```python
from build123d import *

# Parameters (mm, degrees)
SKETCH1_W               = 50
SKETCH1_H               = 100
BOSS_EXTRUDE1_DEPTH     = 90
CUT_EXTRUDE1_DEPTH      = 115.455231423
CUT_EXTRUDE1_DEPTH_BACK = 115.455231423
SKETCH2_R               = 3.2
CHAMFER1_SIZE           = 2
CUT_EXTRUDE2_START      = -5
SKETCH3_W               = 28.111922991
SKETCH3_H               = 15
CUT_EXTRUDE2_DEPTH      = 8
SKETCH4_R               = 4.125
CUT_EXTRUDE3_DEPTH      = 8
SKETCH6_W               = 5
SKETCH6_H               = 5
CUT_EXTRUDE4_DEPTH      = 108.964114408


with BuildPart() as part:
    # Sketch1 → Boss-Extrude1 (new body)
    with BuildSketch(Plane.YZ):
        Rectangle(SKETCH1_W, SKETCH1_H)
    extrude(amount=BOSS_EXTRUDE1_DEPTH)

    # Sketch2 → Cut-Extrude1 (cut, two sides: drawn at the far end of the back side and taken through both)
    with BuildSketch(Plane(origin=(0, 25, 0), x_dir=(-1, 0, 0), z_dir=(0, 1, 0)).offset(-CUT_EXTRUDE1_DEPTH_BACK)):
        with Locations(Location((-15, -25, 0), (0, 0, 90))):
            Circle(SKETCH2_R)
        with Locations(Location((-15, 25, 0), (0, 0, 270))):
            Circle(SKETCH2_R)
    extrude(amount=CUT_EXTRUDE1_DEPTH + CUT_EXTRUDE1_DEPTH_BACK, mode=Mode.SUBTRACT)

    # Chamfer1
    chamfer1_edges = [part.edges().sort_by_distance(p)[0] for p in [
        (45, 25, 50),
        (45, -25, 50),
        (0, 0, 50),
        (90, 0, 50),
        (45, 25, -50),
        (0, 25, 0),
        (90, 25, 0),
        (15, 25, -28.2),
        (15, 25, 28.2),
        (45, -25, -50),
        (15, -25, 28.2),
        (15, -25, -28.2),
        (0, 0, -50),
        (90, 0, -50),
    ]]
    chamfer(chamfer1_edges, length=CHAMFER1_SIZE)

    # Sketch3 → Cut-Extrude2 (cut)
    with BuildSketch(Plane.XY.offset(50).offset(CUT_EXTRUDE2_START)):
        Polygon((66.5, 7.5), (72.995190528, 3.75), (72.995190528, -3.75), (66.5, -7.5), (88, -7.5), (88, 7.5), align=None)
        with Locations((102.055961496, 0)):
            Rectangle(SKETCH3_W, SKETCH3_H)
        Polygon((66.5, -7.5), (72.995190528, -3.75), (72.995190528, 3.75), (66.5, 7.5), (60.004809472, 3.75), (60.004809472, -3.75), align=None)
    cut_extrude2 = extrude(amount=-CUT_EXTRUDE2_DEPTH, mode=Mode.SUBTRACT)

    # Sketch4 → Cut-Extrude3 (cut)
    with BuildSketch(Plane.XY.offset(50)):
        with Locations((66.5, 0)):
            Circle(SKETCH4_R)
    cut_extrude3 = extrude(amount=-CUT_EXTRUDE3_DEPTH, mode=Mode.SUBTRACT)

    # Sketch6 → Cut-Extrude4 (cut, symmetric)
    with BuildSketch(Plane.XZ.offset(-7.5)):
        with Locations((64, 39.5)):
            Rectangle(SKETCH6_W, SKETCH6_H)
    cut_extrude4 = extrude(amount=CUT_EXTRUDE4_DEPTH, both=True, mode=Mode.SUBTRACT)

    # Mirror1: Cut-Extrude2, Cut-Extrude3, Cut-Extrude4 across plane
    add(cut_extrude2.mirror(Plane.XY), mode=Mode.SUBTRACT)
    add(cut_extrude3.mirror(Plane.XY), mode=Mode.SUBTRACT)
    add(cut_extrude4.mirror(Plane.XY), mode=Mode.SUBTRACT)


solid = part.part
```
Build history of the part. All positions in model axes, mm. A direction names the side the tool comes from. Coordinates: 2 decimals unless noted, no trailing zeros. Order: outer loops, then holes, each group sorted by start corner. A loop starts at its lowest first (then second) coordinate and runs counter-clockwise, first axis right, second up. Notation, with made-up numbers: M -36.75,89.25 L -22.75,89.25 A27 cw -22.75,121.25 Z; hole C -29,-29.5 d8. An arc over 180 degrees is marked long. One line per question, with ' | ' between items. Start each with the question number.
1. Tool access for faces 4 (the face through (66.5, -16, -39)), 5 (the face through (62.485, -5.182, 42.834)), 6 (the face through (70.435, 1.239, 47.535)): list every direction of +Z, -Z, +X, -X, +Y, -Y with a clear straight run to the whole face (end or side of a thin tool).
2. Wall check: line 1 along Z through (x, y) = (70.5, -1.5); line 2 along X through (y, z) = (0, -47.85) (3 decimals); line 3 along Y through (x, z) = (69.5, -40.5). Give the ranges that are in metal, low to high. Write a range as [from, to].
3. Cut at C-C (x = 15). Write the cut outline in (y, z), plus the area to 3 significant figures.
4. Cut at A-A (y = 0). Write the cut outline in (x, z) (3 decimals).
5. Flat gauge pins, fed straight in: P1, Ø2, axis at y = 0.5, z = 42.5, coming from the +X side; P2, Ø7.5, axis at x = 66.5, y = 0, coming from the +Z side; P3, Ø7.5, axis at x = 15, z = 25, coming from the -Y side. Where does each tip first touch, or does it go through?
6. Cut at B-B (z = -25). Write the cut outline in (x, y).
7. Mould opens along X. For faces 1 (the face through (61.5, -15, -39)), 2 (the face through (78, 7.5, -41)), 3 (the face through (60.005, 0, -41)) say: +X half, -X half, draft (parallel to the pull), parting line (faces both ways), or undercut.
The answers:
1) face 4: +Y, -Y | face 5: +X | face 6: +Z
2) line 1: z = [-50, -45], [-37, 37], [45, 50] | line 2: x = [0, 62.375], [70.625, 90] | line 3: y = [-25, -7.5], [7.5, 25]
3) outline: M -25,-48 L -23,-50 L 23,-50 L 25,-48 L 25,-30.2 L 23,-28.2 L -23,-28.2 L -25,-30.2 Z; M -25,-19.8 L -23,-21.8 L 23,-21.8 L 25,-19.8 L 25,19.8 L 23,21.8 L -23,21.8 L -25,19.8 Z; M -25,30.2 L -23,28.2 L 23,28.2 L 25,30.2 L 25,48 L 23,50 L -23,50 L -25,48 Z | area: 4,340 mm2
4) outline: M 0,-48 L 2,-50 L 62.375,-50 L 62.375,-45 L 60.005,-45 L 60.005,-37 L 90,-37 L 90,37 L 60.005,37 L 60.005,45 L 62.375,45 L 62.375,50 L 2,50 L 0,48 Z; M 70.625,-50 L 88,-50 L 90,-48 L 90,-45 L 70.625,-45 Z; M 70.625,45 L 90,45 L 90,48 L 88,50 L 70.625,50 Z; hole C 15,-25 d6.4; hole C 15,25 d6.4
5) P1: stops at x = 60 | P2: stops at z = 37 | P3: stops at y = -23.55
6) outline: M 0,-25 L 9.8,-25 L 11.8,-23 L 11.8,23 L 9.8,25 L 2,25 L 0,23 Z; M 18.2,-23 L 20.2,-25 L 90,-25 L 90,23 L 88,25 L 20.2,25 L 18.2,23 Z
7) face 1: undercut | face 2: draft | face 3: +X half
